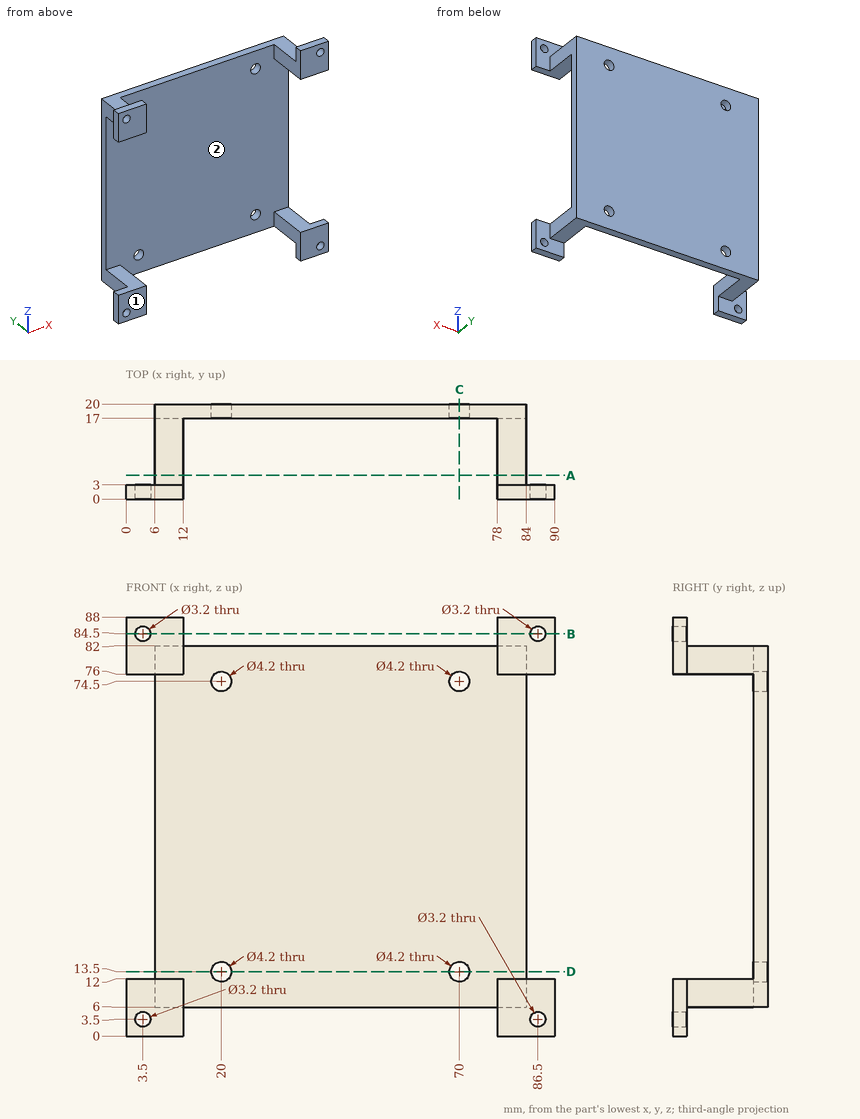
The drawing under review shows one solid part. Ordinate dimensions are in mm from its lowest x, y, z. Give positions to 0.01 mm unless a question says otherwise; leave off trailing zeros. Order: outer loops, then holes, each group sorted by start corner. A loop starts at its lowest first (then second) coordinate and runs counter-clockwise, first axis right, second up. Notation, with made-up numbers: (88.5, 81.25) - (119.5, 81.25) arc R10 ccw to (119.5, 93.25) - close; hole circle Ø2 at (42, -32). An arc over 180 degrees is marked (long way). Answer as a JSON object with one key per item and string values. Group by question number.
Item 1: Draft analysis for pull direction X (two halves, no side actions). For the marked faces 1 and 2, state which applies: pulls with the +X half, pulls with the -X half, needs draft (parallel to the pull), parting line crosses it, or undercut.
Item 2: Take a section at B-B on z = 84.5. Give the boundary of the cut face in (x, y), and give its area (3 significant figures).
Item 3: Take a section at D-D on z = 13.5. Give the boundary of the cut face in (x, y), and give its area (3 significant figures).
Item 4: Take a section at C-C on x = 70. Give the boundary of the cut face in (y, z).
Item 5: Clearance check with flat-ended pins moving along their axes: pin 1 Ø6 at (x, y) = (6.5, 9) entering from -Z; pin 2 Ø5 at (x, z) = (86.5, 84.5) entering from +Y; pin 3 Ø1 at (x, z) = (60, 68) entering from -Y. State where each tip first meets the part, or that it passes through.
Item 6: Wall thickness on line 1 along X through (y, z) = (18.4, 74.5); line 2 along X through (y, z) = (1.6, 84.5); line 3 along Z through (x, y) = (20, 17.8): over which ranges is each line inside the solid? List them lowest first.
Item 7: Take a section at A-A on y = 5. Give the boundary of the cut face in (x, z), and give its area (3 significant figures).
Reported:
{
 "1": {"face 1": "needs draft", "face 2": "undercut"},
 "2": {"outline": "(0, 0) - (1.9, 0) - (1.9, 3) - (0, 3) - close; (5.1, 0) - (12, 0) - (12, 3) - (5.1, 3) - close; (78, 0) - (84.9, 0) - (84.9, 3) - (78, 3) - close; (88.1, 0) - (90, 0) - (90, 3) - (88.1, 3) - close", "area": "52.8 mm^2"},
 "3": {"outline": "(6, 17) - (17.9, 17) - (17.9, 20) - (6, 20) - close; (22.1, 17) - (67.9, 17) - (67.9, 20) - (22.1, 20) - close; (72.1, 17) - (84, 17) - (84, 20) - (72.1, 20) - close", "area": "209 mm^2"},
 "4": {"outline": "(17, 6) - (20, 6) - (20, 11.4) - (17, 11.4) - close; (17, 15.6) - (20, 15.6) - (20, 72.4) - (17, 72.4) - close; (17, 76.6) - (20, 76.6) - (20, 82) - (17, 82) - close"},
 "5": {"pin 1": "z = 6", "pin 2": "y = 3", "pin 3": "y = 17"},
 "6": {"line 1": "6 to 17.9, 22.1 to 67.9, 72.1 to 84", "line 2": "0 to 1.9, 5.1 to 12, 78 to 84.9, 88.1 to 90", "line 3": "6 to 11.4, 15.6 to 72.4, 76.6 to 82"},
 "7": {"outline": "(6, 6) - (12, 6) - (12, 12) - (6, 12) - close; (6, 76) - (12, 76) - (12, 82) - (6, 82) - close; (78, 6) - (84, 6) - (84, 12) - (78, 12) - close; (78, 76) - (84, 76) - (84, 82) - (78, 82) - close", "area": "144 mm^2"}
}
